CAD build for the part. Positions are in the model's coordinates, mm. Face numbers are marked on the shaded views. A direction names the side the tool comes from. Give positions to 0.01 mm unless a question says otherwise; leave off trailing zeros. Write each loop counter-clockwise with the first axis right and the second up, starting at its lowest first coordinate (ties: lowest second). Pieces come first, ordered by that corner, then holes. Notation, with made-up numbers: (58, 52) - (87, 52) arc R32 cw to (87, 82) - close; hole circle Ø5 at (27, -27.5). An arc over 180 degrees is marked (long way). Answer as a JSON object with one key per item and string values.
from build123d import *

# Parameters (mm, degrees)
BOSS_EXTRUDE1_DEPTH    = 52
SKETCH5_W              = 6
SKETCH5_H              = 52
BOSS_BOTTOMALIGN_DEPTH = 0.5
FILLET1_SIZE           = 0.2
CUT_BOTTOMHOLE_REACH   = 57.545
SKETCH3_R              = 1.6
SKETCH7_R              = 2.875
CUT_EXTRUDE6_DEPTH     = 0.4
SKETCH6_R              = 3
CUT_MAGNET_DEPTH       = 3
CUT_EXTRUDE7_REACH     = 56.489
SKETCH8_W              = 28.374522614
SKETCH8_H              = 8
FILLET2_R              = 4
FILLET3_R              = 4


with BuildPart() as part:
    # Sketch1 → Boss-Extrude1 (new body)
    with BuildSketch(Plane.XY):
        Polygon((0, 0), (0, 12), (4, 12), (4, 4), (15, 4), (15, 0), align=None)
    extrude(amount=BOSS_EXTRUDE1_DEPTH)

    # Sketch5 → Boss-BottomAlign (add)
    with BuildSketch(Plane.XZ):
        with Locations((5, 26)):
            Rectangle(SKETCH5_W, SKETCH5_H)
    extrude(amount=BOSS_BOTTOMALIGN_DEPTH)

    # Fillet1
    fillet1_edges = [part.edges().sort_by_distance(p)[0] for p in [
        (8, -0.5, 26),
        (2, -0.5, 26),
    ]]
    chamfer(fillet1_edges, length=FILLET1_SIZE)

    # Sketch3 → Cut-BottomHole (cut, up to next)
    with BuildSketch(Plane.XZ.offset(0.5), mode=Mode.PRIVATE) as cut_bottomhole_sk1:
        with Locations(Location((5, 36, 0), (0, 0, 270))):
            Circle(SKETCH3_R)
    cut_bottomhole_tool1 = extrude(cut_bottomhole_sk1.sketch, amount=-CUT_BOTTOMHOLE_REACH, mode=Mode.PRIVATE) & part.part
    # Sketch3 → Cut-BottomHole (cut, up to next)
    with BuildSketch(Plane.XZ.offset(0.5), mode=Mode.PRIVATE) as cut_bottomhole_sk2:
        with Locations(Location((5, 16, 0), (0, 0, 231.317812547))):
            Circle(SKETCH3_R)
    cut_bottomhole_tool2 = extrude(cut_bottomhole_sk2.sketch, amount=-CUT_BOTTOMHOLE_REACH, mode=Mode.PRIVATE) & part.part
    add(cut_bottomhole_tool1.solids().sort_by_distance((5, -0.5, 36))[0], mode=Mode.SUBTRACT)
    add(cut_bottomhole_tool2.solids().sort_by_distance((5, -0.5, 16))[0], mode=Mode.SUBTRACT)

    # Sketch7 → Cut-Extrude6 (cut)
    with BuildSketch(Plane(origin=(0, 4, 0), x_dir=(1, 0, 0), z_dir=(0, 1, 0))):
        with Locations(Location((5, -36, 0), (0, 0, 270))):
            Circle(SKETCH7_R)
        with Locations(Location((5, -16, 0), (0, 0, 270))):
            Circle(SKETCH7_R)
    extrude(amount=-CUT_EXTRUDE6_DEPTH, mode=Mode.SUBTRACT)

    # Sketch6 → Cut-Magnet (cut)
    with BuildSketch(Plane.ZY):
        with Locations((6, 6)):
            Circle(SKETCH6_R)
        with Locations(Location((46, 6, 0), (0, 0, 180))):
            Circle(SKETCH6_R)
    extrude(amount=-CUT_MAGNET_DEPTH, mode=Mode.SUBTRACT)

    # Sketch8 → Cut-Extrude7 (cut, up to next)
    with BuildSketch(Plane(origin=(4, 0, 0), x_dir=(0, 0, -1), z_dir=(1, 0, 0)), mode=Mode.PRIVATE) as cut_extrude7_sk1:
        with Locations((-25.812738693, 8)):
            Rectangle(SKETCH8_W, SKETCH8_H)
    cut_extrude7_tool1 = extrude(cut_extrude7_sk1.sketch, amount=-CUT_EXTRUDE7_REACH, mode=Mode.PRIVATE) & part.part
    add(cut_extrude7_tool1.solids().sort_by_distance((4, 8, 25.812739))[0], mode=Mode.SUBTRACT)

    # Fillet2
    fillet2_edges = [part.edges().sort_by_distance(p)[0] for p in [
        (2, 12, 11.625477386),
        (2, 12, 40),
        (2, 12, 52),
        (2, 12, 0),
    ]]
    fillet(fillet2_edges, radius=FILLET2_R)

    # Fillet3
    fillet3_edges = [part.edges().sort_by_distance(p)[0] for p in [
        (15, 2, 0),
        (15, 2, 52),
    ]]
    fillet(fillet3_edges, radius=FILLET3_R)


solid = part.part
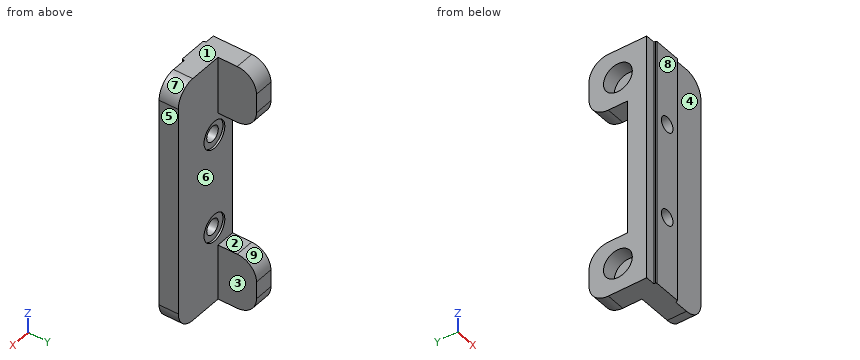
Item 1: Flat gauge pins, fed straight in: P1, Ø1, axis at x = 1, z = 36, coming from the -Y side; P2, Ø4.5, axis at x = 5, z = 36, coming from the +Y side; P3, Ø3, axis at x = 6.5, z = 16.5, coming from the +Y side. Where does each tip first touch, or does it go through?
Entries:
{"P1": "y = 0", "P2": "y = 3.6", "P3": "y = 4"}
Item 2: Probe line 1 (Z direction, x = 5, y = 3.8) (3 decimals); line 2 (X direction, y = 0.9, z = 16); line 3 (X direction, y = 3.95, z = 36) (3 decimals). List the from-to ranges inside material, lowest first. Write a range as from..to.
Entries:
{"line 1": "0..13.125, 18.875..33.125, 38.875..52", "line 2": "0..3.4, 6.6..15", "line 3": "0..2.125, 7.875..15"}
Item 3: Cut at B-B (z = 36). Give the cut face in (x, y) (3 decimals).
Entries:
{"outline": "(0, 0) - (2, 0) - (2, -0.3) - (2.2, -0.5) - (3.4, -0.5) - (3.4, 3.6) - (2.125, 3.6) - (2.125, 4) - (0, 4) - close; (6.6, -0.5) - (7.8, -0.5) - (8, -0.3) - (8, 0) - (15, 0) - (15, 4) - (7.875, 4) - (7.875, 3.6) - (6.6, 3.6) - close"}
Item 4: Cut at C-C (y = 6). Give the cut face in (x, z).
Entries:
{"outline": "(0, 0) - (4, 0) - (4, 11.63) - (0, 11.63) - (0, 9) - (3, 9) - (3, 3) - (0, 3) - close; (0, 40) - (4, 40) - (4, 52) - (0, 52) - (0, 49) - (3, 49) - (3, 43) - (0, 43) - close"}
Item 5: Mould opens along Z. For the marked faces 6, 7, 8 and 9 say: +Z half, -Z half, draft (parallel to the pull), parting line (faces both ways), or undercut.
Entries:
{"face 6": "undercut", "face 7": "+Z half", "face 8": "draft", "face 9": "undercut"}
Item 6: Which spindle directions (+Z, -Z, +X, -X, +Y, -Y) get a long thin tool onto all of the face, cutting with end or side? Do the marked faces 1, 2, 3, 4 and 5. Say none if no direction does.
Entries:
{"face 1": "+Z, +X, -X, +Y, -Y", "face 2": "+X, -X, +Y", "face 3": "+Z, -Z, +X, +Y", "face 4": "+Z, -Z, +X, -Y", "face 5": "+Z, -Z, +X, +Y, -Y"}
Item 7: Cut at D-D (z = 46). Give the cut face in (x, y).
Entries:
{"outline": "(0, 0) - (2, 0) - (2, -0.3) - (2.2, -0.5) - (7.8, -0.5) - (8, -0.3) - (8, 0) - (15, 0) - (15, 4) - (4, 4) - (4, 12) - (0, 12) - (0, 9) - (3, 9) - (3, 3) - (0, 3) - close"}
Item 8: Cut at A-A (x = 5). Give the cut face in (y, z) (3 decimals), and give its area (3 significant figures).
Entries:
{"outline": "(-0.5, 0) - (4, 0) - (4, 13.125) - (3.6, 13.125) - (3.6, 14.4) - (-0.5, 14.4) - close; (-0.5, 17.6) - (3.6, 17.6) - (3.6, 18.875) - (4, 18.875) - (4, 33.125) - (3.6, 33.125) - (3.6, 34.4) - (-0.5, 34.4) - close; (-0.5, 37.6) - (3.6, 37.6) - (3.6, 38.875) - (4, 38.875) - (4, 52) - (-0.5, 52) - close", "area": "203 mm2"}
